Could you check a few things on this model? Use its own coordinates, in mm. A direction names the side the tool comes from. Coordinates: 2 decimals unless noted, no trailing zeros. Order: outer loops, then holes, each group sorted by start corner. A loop starts at its lowest first (then second) coordinate and runs counter-clockwise, first axis right, second up. Notation, with made-up numbers: (78, 78) - (124, 78) arc R22 ccw to (124, 85) - close; hole circle Ø9 at (-3.75, 8.25). An arc over 180 degrees is marked (long way). Answer as CSV lines item,"result". Start each with the question number.
1. I need wall thicknesses on probe 1 along Z at (x, y) = (-3.5, -3); probe 2 along Z at (x, y) = (-0.25, -0.5); probe 3 along Y at (x, z) = (-1.25, -3.25). Which ranges of each line are inside material? Lowest first, please.
2. For faces 1 (the face through (-2.54, 0, -4)), 2 (the face through (2, -2, -6.35)), which set-ups out of +Z, -Z, +X, -X, +Y, -Y let a thin tool reach every point of the face, with its end or its side?
3. Thinking about a two-plate mould opening in Y: for faces 3 (the face through (0, 0, 12.7)), 4 (the face through (-0.69, -3.1, 6.01)), 5 (the face through (1.25, 2.21, -4.47)), which applies, released by +Y, released by -Y, zero draft, split by the parting line, or undercut?
4. I want a section at C-C, the plane z = -1.25. List the corners of the cut face in (x, y) for me (1 decimal), and give its area (3 significant figures).
5. I want a section at B-B, the plane z = 9. List the corners of the cut face in (x, y) for me (3 decimals).
6. For pin 1 (1 mm diameter, centred on x = -0.5, z = 0, fed in from -Y); pin 2 (1.5 mm diameter, centred on x = 1, y = -1, fed in from -Z); pin 3 (1.5 mm diameter, centred on x = -2, z = 7.5, fed in from +Y), each with a flat end and sliding along its axis, tell me the tip position at first contact or that it passes through.
7. I want a section at D-D, the plane y = -3.75. List the corners of the cut face in (x, z) for me.
from build123d import *

# Parameters (mm, degrees)
SKETCH1_R           = 4.7625
BOSS_EXTRUDE1_DEPTH = 6.35
SKETCH2_R           = 3.175
BOSS_EXTRUDE2_DEPTH = 12.7
CHAMFER1_SIZE       = 0.508
CUT_EXTRUDE1_DEPTH  = 3.81


with BuildPart() as part:
    # Sketch1 → Boss-Extrude1 (new body)
    with BuildSketch(Plane.XY):
        Circle(SKETCH1_R)
    extrude(amount=-BOSS_EXTRUDE1_DEPTH)

    # Sketch2 → Boss-Extrude2 (add)
    with BuildSketch(Plane.XY):
        Circle(SKETCH2_R)
    extrude(amount=BOSS_EXTRUDE2_DEPTH)

    # Chamfer1
    chamfer1_edges = [part.edges().sort_by_distance(p)[0] for p in [
        (-3.175, 0, 12.7),
    ]]
    chamfer(chamfer1_edges, length=CHAMFER1_SIZE)

    # Sketch3 → Cut-Extrude1 (cut)
    with BuildSketch(Plane(origin=(0, 0, -6.35), x_dir=(-1, 0, 0), z_dir=(0, 0, -1))):
        Polygon((0, 2.932939367), (-2.54, 1.466469684), (-2.54, -1.466469684), (0, -2.932939367), (2.54, -1.466469684), (2.54, 1.466469684), align=None)
    extrude(amount=-CUT_EXTRUDE1_DEPTH, mode=Mode.SUBTRACT)


solid = part.part
Solved:
1,probe 1,"z = -6.35 to 0"
1,probe 2,"z = -2.54 to 12.7"
1,probe 3,"y = -4.6 to -2.21, 2.21 to 4.6"
2,face 1,"-Z"
2,face 2,"-Z, +X, -X, +Y, -Y"
3,face 3,"zero draft"
3,face 4,"split by the parting line"
3,face 5,"undercut"
4,outline,"circle Ø9.5 at (0, 0)"
4,area,"71.3 mm2"
5,outline,"circle Ø6.35 at (0, 0)"
6,pin 1,"stops at y = -4.76"
6,pin 2,"stops at z = -2.54"
6,pin 3,"stops at y = 2.92"
7,outline,"(-2.94, -6.35) - (2.94, -6.35) - (2.94, 0) - (-2.94, 0) - close"
